Read the model definition and answer for the solid it produces. Units are mm, in the model's axes. Round coordinates to 2 decimals unless told otherwise and drop trailing zeros. Order: outer loops, then holes, each group sorted by start corner. A loop starts at its lowest first (then second) coordinate and runs counter-clockwise, first axis right, second up. Notation, with made-up numbers: (33, -31) -> (67, -31) arc R11 cw to (67, -26) -> close; hole circle Ø4 at (-36.5, 24). An arc over 180 degrees is marked (long way). Answer as a JSON object with one key per item and string values. Group by question number.
Item 1: Consider probe 1 along X at (y, z) = (8.25, 1); probe 2 along Z at (x, y) = (8, -10.25); probe 3 along Y at (x, z) = (4.5, 1). Determine where each line is inside the solid, lowest interval first. Write a range as from..to.
Item 2: Section B-B, the plane y = 1.25 is taken. Write down the section's boundary in (x, z).
Item 3: Section C-C, the plane x = 10.75 is taken. Write down the section's boundary in (y, z), plus the area to 3 significant figures.
Item 4: Given P1, Ø1, axis at x = 3.5, y = -7.5, coming from the -Z side, flat-ended and moving along its own axis, determine where the tip first touches the part or whether it passes through.
Item 5: Section A-A, the plane z = 21.5 is taken. Write down the section's boundary in (x, y).
from build123d import *

# Parameters (mm, degrees)
F0_W     = 24.954888
F0_H     = 48.623441
F1_DEPTH = 12.7
F2_R     = 5.08
F3_SIZE  = 5.08


with BuildPart() as f1:
    # F0 (on Right) → F1 (new body)
    with BuildSketch(Plane.YZ):
        with Locations((-3.215835, 9.647509)):
            Rectangle(F0_W, F0_H)
    extrude(amount=F1_DEPTH)

    # F2
    f2_edges = [f1.edges().sort_by_distance(p)[0] for p in [
        (6.35, -15.693279, -14.664212),
        (6.35, 9.261609, -14.664212),
    ]]
    fillet(f2_edges, radius=F2_R)

    # F3
    f3_edges = [f1.edges().sort_by_distance(p)[0] for p in [
        (12.7, -3.215835, -14.664212),
        (0, -3.215835, -14.664212),
    ]]
    chamfer(f3_edges, length=F3_SIZE)


solid = f1.part
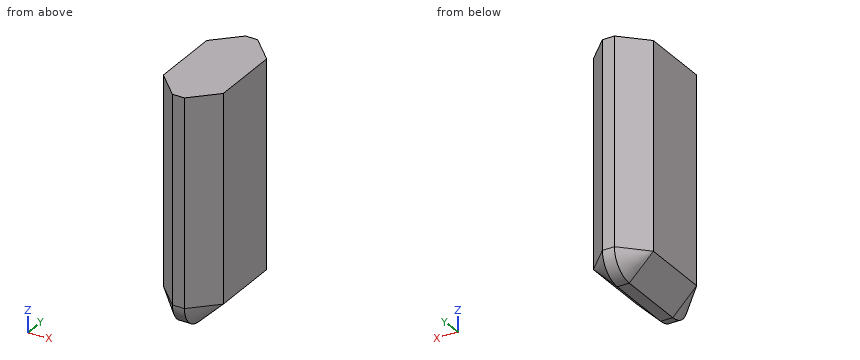
Values found:
{
 "1": {"probe 1": "4.07..8.63", "probe 2": "-14.28..33.96", "probe 3": "-15.11..8.68"},
 "2": {"outline": "(0, -9.58) -> (5.08, -14.66) -> (7.62, -14.66) -> (12.7, -9.58) -> (12.7, 33.96) -> (0, 33.96) -> close"},
 "3": {"outline": "(-12.56, -9.58) arc R1.95 ccw to (-10.61, -11.53) -> (4.18, -11.53) arc R1.95 ccw to (6.13, -9.58) -> (6.13, 33.96) -> (-12.56, 33.96) -> close", "area": "849 mm2"},
 "4": {"P1": "z = -13.58"},
 "5": {"outline": "(0, -10.61) -> (5.08, -15.69) -> (7.62, -15.69) -> (12.7, -10.61) -> (12.7, 4.18) -> (7.62, 9.26) -> (5.08, 9.26) -> (0, 4.18) -> close"}
}
